Here's how the part is built. I have some questions about the finished solid (model axes, mm). A direction names the side the tool comes from. Coordinates: 2 decimals unless noted, no trailing zeros. Order: outer loops, then holes, each group sorted by start corner. A loop starts at its lowest first (then second) coordinate and runs counter-clockwise, first axis right, second up. Notation, with made-up numbers: (46.5, 35) - (74.5, 35) arc R27 ccw to (74.5, 70) - close; hole circle Ø5 at (-5.75, 33). An arc over 180 degrees is marked (long way). Answer as CSV lines item,"result". Start each with the question number.
Q1. For pin 1 Ø1.3 at (x, z) = (367, -127.5) entering from +Y; pin 2 Ø4 at (x, y) = (-321.5, 269.5) entering from +Z; pin 3 Ø12 at (y, z) = (36.5, 271.5) entering from -X; pin 4 Ø15 at (y, z) = (305, -24) entering from -X, each with a flat end and sliding along its axis, tell me the tip position at first contact or that it passes through.
Q2. For faces 4 (the face through (301.062, 231.763, 424.212)), 5 (the face through (306, 254, 580)), which set-ups out of +Z, -Z, +X, -X, +Y, -Y let a thin tool reach every point of the face, with its end or its side?
Q3. I need wall thicknesses on line 1 (Y direction, x = 86.5, z = -326); line 2 (Z direction, x = -329, y = 55); line 3 (Z direction, x = 65, y = 115). Which ranges of each line are inside material? Lowest first, please.
Q4. Suppose I cut it at A-A (y = 51.5). Please give me the cut outline in (x, z), then the cut area to 3 significant figures.
Q5. Suppose I cut it at B-B (z = 300). Please give me the cut outline in (x, y), then the cut area to 3 significant figures.
Q6. Thinking about a two-plate mould opening in Z: for faces 1 (the face through (265.33, 255.1, -417.4)), 2 (the face through (5, 143, 264)), 3 (the face through (4, 290, -344)), which applies, released by +Z, released by -Z, zero draft, split by the parting line, or undercut?
Q7. Suppose I cut it at C-C (z = -284). Please give me the cut outline in (x, y).
from build123d import *

# Parameters (mm, degrees)
EXTRUDE_1_DEPTH     = 320
EXTRUDE_2_DEPTH     = 30
CUT_EXTRUDE_1_DEPTH = 30
SKETCH_4_R          = 25
EXTRUDE_3_DEPTH     = 580
EXTRUDE_3_TAPER     = 0.3
SKETCH_8_R          = 25
EXTRUDE_4_DEPTH     = 557.556275
SKETCH_9_R          = 25
EXTRUDE_5_DEPTH     = 585.675678


with BuildPart() as part:
    # 草图1 → 凸台-拉伸1 (new body)
    with BuildSketch(Plane(origin=(0, 0, 0), x_dir=(1, 0, 0), z_dir=(0, 1, 0))):
        Polygon((368, -264), (-368, -264), (-367, 301), (368.6, 303.3), align=None)
    extrude(amount=EXTRUDE_1_DEPTH)

    # 草图2 → 凸台-拉伸2 (add)
    with BuildSketch(Plane(origin=(0, 320, 0), x_dir=(1, 0, 0), z_dir=(0, 1, 0))):
        Polygon((363.5, 385), (370, -383), (-365.5, -384), (-365.8, 384.5), align=None)
    extrude(amount=-EXTRUDE_2_DEPTH)

    # 草图3 → 切除-拉伸1 (cut)
    with BuildSketch(Plane(origin=(0, 320, 0), x_dir=(1, 0, 0), z_dir=(0, 1, 0))):
        Polygon((364.191588014, 303.286216221), (368.110287471, -159.723196528), (368.6, 303.3), align=None)
        Polygon((-365.767405538, 301.003853952), (-365.546844502, -264), (-368, -264), (-367, 301), align=None)
    extrude(amount=-CUT_EXTRUDE_1_DEPTH, mode=Mode.SUBTRACT)

    # 草图4 → 凸台-拉伸3 (add)
    with BuildSketch(Plane.XY):
        with Locations((306, 254)):
            Circle(SKETCH_4_R)
    extrude(amount=EXTRUDE_3_DEPTH, taper=EXTRUDE_3_TAPER)

    # 草图8 → 凸台-拉伸4 (add)
    with BuildSketch(Plane(origin=(0, 254, -300), x_dir=(0.26903113941240836, 0, -0.9631314790964218), z_dir=(0.9631314790964218, 0, 0.26903113941240836))):
        Circle(SKETCH_8_R)
    extrude(amount=-EXTRUDE_4_DEPTH)

    # 草图9 → 凸台-拉伸5 (add)
    with BuildSketch(Plane(origin=(0, 254, -300), x_dir=(0.3244116275984733, 0, 0.9459160088923908), z_dir=(-0.9459160088923909, 0, 0.3244116275984733))):
        Circle(SKETCH_9_R)
    extrude(amount=-EXTRUDE_5_DEPTH)


solid = part.part
Here are the results:
1,pin 1,"stops at y = 290"
1,pin 2,"stops at z = 264"
1,pin 3,"passes through"
1,pin 4,"stops at x = -365.66"
2,face 4,"+Z"
2,face 5,"+Z, +X, -X, +Y, -Y"
3,line 1,"y = 229.24 to 278.76, 290 to 320"
3,line 2,"z = -301.12 to 264"
3,line 3,"z = -302.35 to 264"
4,outline,"(-368, 264) - (-367, -301) - (368.6, -303.3) - (368, 264) - close"
4,area,"417,000 mm²"
5,outline,"(-365.53, 290) - (369.3, 290) - (369.3, 320) - (-365.53, 320) - close; circle Ø46.86 at (306, 254)"
5,area,"23,800 mm²"
6,face 1,"undercut"
6,face 2,"released by +Z"
6,face 3,"zero draft"
7,outline,"(-367.03, 0) - (368.58, 0) - (368.58, 290) - (364.35, 290) - (364.35, 320) - (-365.76, 320) - (-365.76, 290) - (-367.03, 290) - close"
